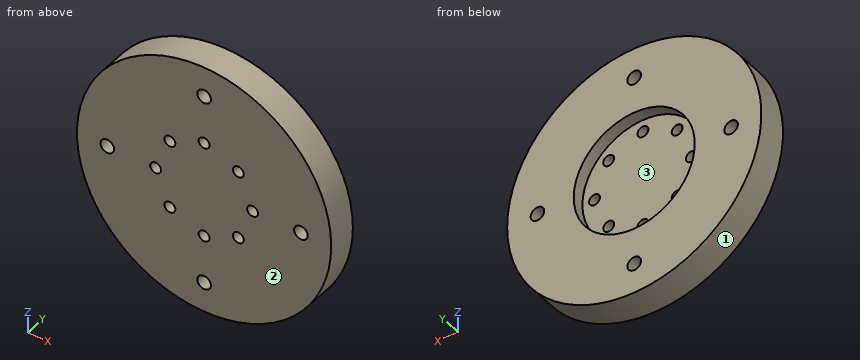
```python
from build123d import *

# Parameters (mm, degrees)
SKETCH_1_R          = 21
EXTRUDE_1_DEPTH     = 5
SKETCH_2_R          = 10
CUT_EXTRUDE_1_DEPTH = 2
SKETCH_3_R          = 0.9
CUT_EXTRUDE_2_DEPTH = 3
SKETCH_4_R          = 1.125
CUT_EXTRUDE_3_DEPTH = 5


with BuildPart() as part:
    # 스케치1 → 보스-돌출1 (new body)
    with BuildSketch(Plane(origin=(0, 0, 0), x_dir=(1, 0, 0), z_dir=(0, 1, 0))):
        Circle(SKETCH_1_R)
    extrude(amount=EXTRUDE_1_DEPTH)

    # 스케치2 → 컷-돌출1 (cut)
    with BuildSketch(Plane(origin=(0, 5, 0), x_dir=(1, 0, 0), z_dir=(0, 1, 0))):
        Circle(SKETCH_2_R)
    extrude(amount=-CUT_EXTRUDE_1_DEPTH, mode=Mode.SUBTRACT)

    # 스케치3 → 컷-돌출2 (cut)
    with BuildSketch(Plane(origin=(0, 3, 0), x_dir=(1, 0, 0), z_dir=(0, 1, 0))):
        with Locations((5.656854249, 5.656854249)):
            Circle(SKETCH_3_R)
        with Locations((8, 0)):
            Circle(SKETCH_3_R)
        with Locations((0, 8)):
            Circle(SKETCH_3_R)
        with Locations((5.656854249, -5.656854249)):
            Circle(SKETCH_3_R)
        with Locations((0, -8)):
            Circle(SKETCH_3_R)
        with Locations((-5.656854249, -5.656854249)):
            Circle(SKETCH_3_R)
        with Locations((-8, 0)):
            Circle(SKETCH_3_R)
        with Locations((-5.656854249, 5.656854249)):
            Circle(SKETCH_3_R)
    extrude(amount=-CUT_EXTRUDE_2_DEPTH, mode=Mode.SUBTRACT)

    # 스케치4 → 컷-돌출3 (cut)
    with BuildSketch(Plane.XZ):
        with Locations((0, -16)):
            Circle(SKETCH_4_R)
        with Locations((-16, 0)):
            Circle(SKETCH_4_R)
        with Locations((0, 16)):
            Circle(SKETCH_4_R)
        with Locations((16, 0)):
            Circle(SKETCH_4_R)
    extrude(amount=-CUT_EXTRUDE_3_DEPTH, mode=Mode.SUBTRACT)


solid = part.part
```
Check sheet for the modelled part. Datum: model origin and axes. Units: mm. Face numbers are marked on the shaded views. Give positions to 0.01 mm unless a question says otherwise; leave off trailing zeros. Order: outer loops, then holes, each group sorted by start corner. A loop starts at its lowest first (then second) coordinate and runs counter-clockwise, first axis right, second up. Notation, with made-up numbers: M 30,16 L 53,16 A15 ccw 53,39 Z; hole C 34.25,21 d5. An arc over 180 degrees is marked long. Answer in a Markdown table with one row per item.
1) Cross-section at A-A, the plane x = 0. Enter the section's corners in (y, z) (3 decimals).
Filled sheet:
| item | result |
|---|---|
| outline | M 0,-21 L 5,-21 L 5,-17.125 L 0,-17.125 Z; M 0,-14.875 L 5,-14.875 L 5,-10 L 3,-10 L 3,-8.9 L 0,-8.9 Z; M 0,-7.1 L 3,-7.1 L 3,7.1 L 0,7.1 Z; M 0,8.9 L 3,8.9 L 3,10 L 5,10 L 5,14.875 L 0,14.875 Z; M 0,17.125 L 5,17.125 L 5,21 L 0,21 Z |
2) Gauge pin test, flat ends, axial feed: P1, Ø1, axis at y = 4, z = -5.5, coming from the -X side; P2, Ø2, axis at x = 12.5, y = 4, coming from the +Z side; P3, Ø1.5, axis at y = 2, z = -12, coming from the +X side. Record the tip position at first contact, or that the pin passes through.
Filled sheet:
| item | result |
|---|---|
| P1 | stops at x = -20.4 |
| P2 | stops at z = 17.57 |
| P3 | stops at x = 17.73 |
3) Release check for a two-part mould opening along Z. For the marked faces 1, 2 and 3 record: +Z half, -Z half, draft (parallel to the pull), parting line (faces both ways), or undercut.
Filled sheet:
| item | result |
|---|---|
| face 1 | parting line |
| face 2 | draft |
| face 3 | undercut |
4) Thickness scan on L1, parallel to Z at x = 0, y = 2.35 (3 decimals); L2, parallel to Z at x = 0, y = 3.25 (3 decimals); L3, parallel to Z at x = 8.5, y = 0.4. Record the ranges inside material, lowest first. Write a range as [from, to].
Filled sheet:
| item | result |
|---|---|
| L1 | z = [-21, -17.125], [-14.875, -8.9], [-7.1, 7.1], [8.9, 14.875], [17.125, 21] |
| L2 | z = [-21, -17.125], [-14.875, -10], [10, 14.875], [17.125, 21] |
| L3 | z = [-19.2, -0.75], [0.75, 19.2] |
5) Cross-section at D-D, the plane x = 8. Enter the section's corners in (y, z).
Filled sheet:
| item | result |
|---|---|
| outline | M 0,-19.42 L 5,-19.42 L 5,-6 L 3,-6 L 3,-0.9 L 0,-0.9 Z; M 0,0.9 L 3,0.9 L 3,6 L 5,6 L 5,19.42 L 0,19.42 Z |
6) Cross-section at B-B, the plane z = 0. Enter the section's corners in (x, y) (3 decimals), plus the area to 3 significant figures.
Filled sheet:
| item | result |
|---|---|
| outline | M -21,0 L -17.125,0 L -17.125,5 L -21,5 Z; M -14.875,0 L -8.9,0 L -8.9,3 L -10,3 L -10,5 L -14.875,5 Z; M -7.1,0 L 7.1,0 L 7.1,3 L -7.1,3 Z; M 8.9,0 L 14.875,0 L 14.875,5 L 10,5 L 10,3 L 8.9,3 Z; M 17.125,0 L 21,0 L 21,5 L 17.125,5 Z |
| area | 137 mm2 |
7) Cross-section at C-C, the plane y = 4.1. Enter the section's corners in (x, z) (3 decimals), plus the area to 3 significant figures.
Filled sheet:
| item | result |
|---|---|
| outline | C 0,0 d42; hole C -16,0 d2.25; hole C 0,0 d20; hole C 0,-16 d2.25; hole C 0,16 d2.25; hole C 16,0 d2.25 |
| area | 1,060 mm2 |
